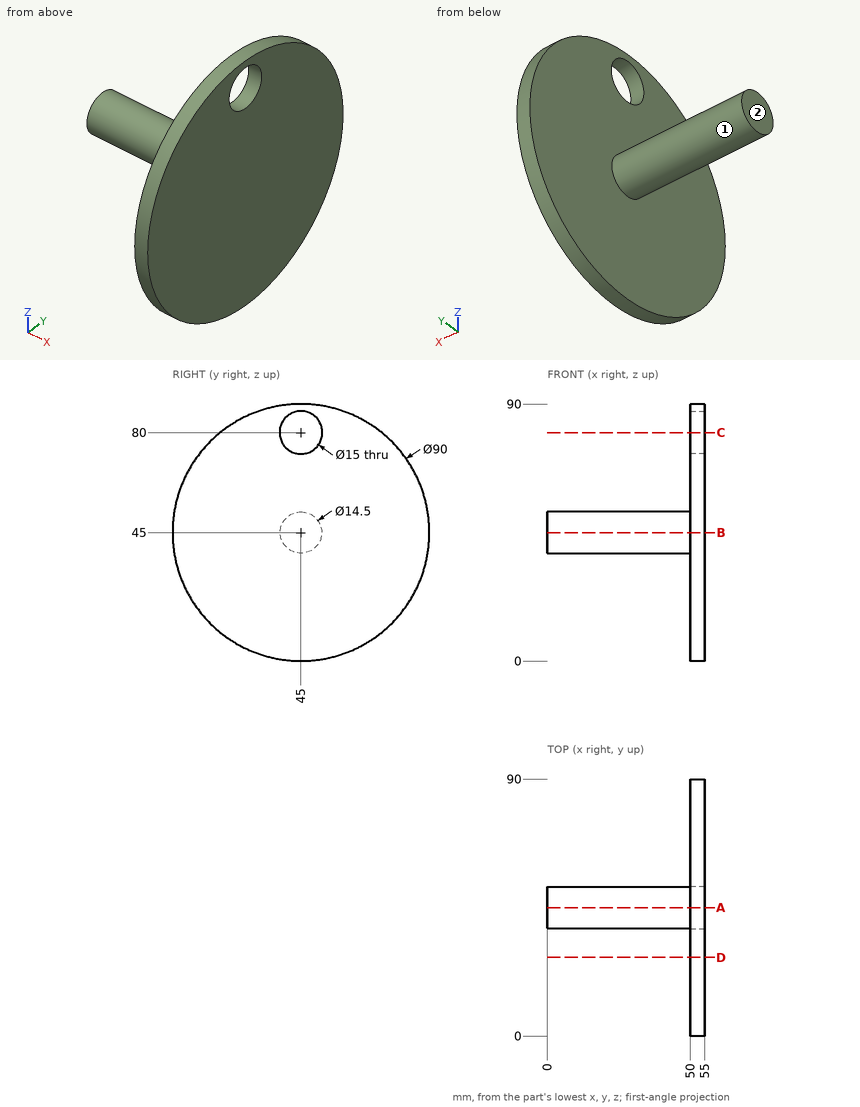
Drawing for the job (mm, zero at the part's lowest x, y, z). A direction names the side the tool comes from. Coordinates: 2 decimals unless noted, no trailing zeros. Order: outer loops, then holes, each group sorted by start corner. A loop starts at its lowest first (then second) coordinate and runs counter-clockwise, first axis right, second up. Notation, with made-up numbers: (49.5, -31.5) -> (87.5, -31.5) arc R9 ccw to (87.5, -17.5) -> close; hole circle Ø8 at (81.5, -30). An arc over 180 degrees is marked (long way). Return JSON: item names as keys, results as strings.
Item 1: Slice it at A-A (y = 45). Write the cut outline in (x, z), then the cut area to 3 significant figures.
Model answer:
{"outline": "(0, 37.75) -> (50, 37.75) -> (50, 0) -> (55, 0) -> (55, 72.5) -> (50, 72.5) -> (50, 52.25) -> (0, 52.25) -> close; (50, 87.5) -> (55, 87.5) -> (55, 90) -> (50, 90) -> close", "area": "1,100 mm²"}
Item 2: Slice it at C-C (z = 80). Write the cut outline in (x, y), then the cut area to 3 significant figures.
Model answer:
{"outline": "(50, 16.72) -> (55, 16.72) -> (55, 37.5) -> (50, 37.5) -> close; (50, 52.5) -> (55, 52.5) -> (55, 73.28) -> (50, 73.28) -> close", "area": "208 mm²"}
Item 3: Wall check: line 1 along X through (y, z) = (55.5, 30); line 2 along Y through (x, z) = (53.15, 80); line 3 along Z through (x, y) = (38, 49). Give the ranges that are in metal, low to high. Write a range as from..to.
Model answer:
{"line 1": "x = 50..55", "line 2": "y = 16.72..37.5, 52.5..73.28", "line 3": "z = 38.95..51.05"}
Item 4: Slice it at B-B (z = 45). Write the cut outline in (x, y).
Model answer:
{"outline": "(0, 37.75) -> (50, 37.75) -> (50, 0) -> (55, 0) -> (55, 90) -> (50, 90) -> (50, 52.25) -> (0, 52.25) -> close"}
Item 5: Pin check, flat tips, straight feed: P1, Ø8, axis at y = 52, z = 63, coming from the -X side; P2, Ø5, axis at x = 25.5, z = 50.5, coming from the -Y side. Stop position of each tip, or through.
Model answer:
{"P1": "stops at x = 50", "P2": "stops at y = 38.4"}
Item 6: Slice it at D-D (y = 27.5). Write the cut outline in (x, z).
Model answer:
{"outline": "(50, 3.54) -> (55, 3.54) -> (55, 86.46) -> (50, 86.46) -> close"}
Item 7: 3-axis set-ups, long thin cutter, end or side, ignore diameter. For the marked faces 1 and 2: which of +Z, -Z, +X, -X, +Y, -Y reach the whole face in a straight line?
Model answer:
{"face 1": "-X", "face 2": "+Z, -Z, -X, +Y, -Y"}
